CAD build for the part. Positions are in the model's coordinates, mm. A direction names the side the tool comes from. Coordinates: 2 decimals unless noted, no trailing zeros. Order: outer loops, then holes, each group sorted by start corner. A loop starts at its lowest first (then second) coordinate and runs counter-clockwise, first axis right, second up. Notation, with made-up numbers: (24.5, 81.25) - (71.5, 81.25) arc R17 ccw to (71.5, 110.25) - close; hole circle Ø10 at (80, 78.25). An arc over 180 degrees is marked (long way). Write each question's results on one line, items separated by ' | '. Start each with the question number.
Q1. Band-saw the part on B-B, the plane x = 60.5. Write the cut outline in (y, z) (3 decimals).
Q2. Pin check, flat tips, straight feed: P1, Ø1, axis at x = 22, z = 11, coming from the +Y side; P2, Ø2.5, axis at x = -77.08, y = -71.12, coming from the -Z side; P3, Ø6, axis at y = 8.5, z = 13.5, coming from the -X side. Stop position of each tip, or through.
Q3. Pull direction Y, two halves, no side cores. Call faces 5 (the flat face through (-2, 69.215, 9)), 6 (the flat face through (-2, 76.2, 4)), 7 (the flat face through (-2, -69.215, 9)), 8 (the flat face through (133.35, -1, 4)): released by +Y, released by -Y, zero draft, split by the parting line, or undercut.
Q4. Band-saw the part on A-A, the plane y = 1. Write the cut outline in (x, z) (3 decimals), then the cut area to 3 significant figures.
Q5. Wall check: probe 1 along Y at (x, z) = (-26, 6.25) (3 decimals); probe 2 along X at (y, z) = (0.5, 8.25) (3 decimals); probe 3 along Y at (x, z) = (53.5, 6.5) (3 decimals). Give the ranges that are in metal, low to high.
Q6. Which spindle directions (+Z, -Z, +X, -X, +Y, -Y) get a long thin tool onto all of the face, cutting with end or side? Do faces 1 (the flat face through (-2, 73.152, 13)), 2 (the flat face through (-2, -73.152, 13)), 3 (the flat face through (130.302, -1, 13)), 4 (the flat face through (-126.365, -1, 9)). Say none if no direction does.
```python
from build123d import *

# Parameters (mm, degrees)
F0_W      = 266.7
F0_H      = 152.4
F0_W_2    = 252.73
F0_H_2    = 138.43
F1_DEPTH  = 17.78
F2_W      = 266.7
F2_H      = 152.4
F2_W_2    = 260.604
F2_H_2    = 146.304
F3_DEPTH  = 8.89
F4_W      = 263.4996
F4_H      = 149.1996
F4_W_2    = 260.35
F4_H_2    = 146.05
F5_DEPTH  = 1.27
F6_R      = 0.762
F7_R      = 1.905
F8_R      = 1.4986
F9_DEPTH  = 8.128
F10_R     = 1.4224
F11_DEPTH = 25.4


with BuildPart() as f1:
    # F0 (on Top) → F1 (new body)
    with BuildSketch(Plane.XY):
        Rectangle(F0_W, F0_H)
        Rectangle(F0_W_2, F0_H_2, mode=Mode.SUBTRACT)
    extrude(amount=F1_DEPTH)

    # F2 (on face) → F3 (cut)
    with BuildSketch(Plane.XY.offset(17.78)):
        Rectangle(F2_W, F2_H)
        Rectangle(F2_W_2, F2_H_2, mode=Mode.SUBTRACT)
    extrude(amount=-F3_DEPTH, mode=Mode.SUBTRACT)

    # F4 (on face) → F5 (cut)
    with BuildSketch(Plane(origin=(0, 0, 0), x_dir=(1, 0, 0), z_dir=(0, 0, -1))):
        Rectangle(F4_W, F4_H)
        Rectangle(F4_W_2, F4_H_2, mode=Mode.SUBTRACT)
    extrude(amount=-F5_DEPTH, mode=Mode.SUBTRACT)

    # F6
    f6_edges = [f1.edges().sort_by_distance(p)[0] for p in [
        (-126.365, -69.215, 8.89),
        (126.365, -69.215, 8.89),
        (126.365, 69.215, 8.89),
        (-126.365, 69.215, 8.89),
    ]]
    fillet(f6_edges, radius=F6_R)

    # F7
    f7_edges = [f1.edges().sort_by_distance(p)[0] for p in [
        (130.175, 73.025, 0.635),
        (131.7498, 74.5998, 0.635),
        (-130.175, 73.025, 0.635),
        (-131.7498, 74.5998, 0.635),
        (-130.175, -73.025, 0.635),
        (-131.7498, -74.5998, 0.635),
        (130.175, -73.025, 0.635),
        (131.7498, -74.5998, 0.635),
    ]]
    fillet(f7_edges, radius=F7_R)

    # F8 (on face) → F9 (cut)
    with BuildSketch(Plane(origin=(0, 0, 0), x_dir=(1, 0, 0), z_dir=(0, 0, -1))):
        with Locations((127.949095, -71.12)):
            Circle(F8_R)
        with Locations((128.141546, -28.642724)):
            Circle(F8_R)
        with Locations((128.34959, 17.276384)):
            Circle(F8_R)
        with Locations((-127.949095, -71.12)):
            Circle(F8_R)
        with Locations((-128.34959, 17.276384)):
            Circle(F8_R)
        with Locations((-128.141546, -28.642724)):
            Circle(F8_R)
        with Locations((76.691895, -71.12)):
            Circle(F8_R)
        with Locations((25.434695, -71.12)):
            Circle(F8_R)
        with Locations((-25.822505, -71.12)):
            Circle(F8_R)
        with Locations((-77.079705, -71.12)):
            Circle(F8_R)
        with Locations((76.691895, 71.12)):
            Circle(F8_R)
        with Locations((127.949095, 71.12)):
            Circle(F8_R)
        with Locations((-127.949095, 71.12)):
            Circle(F8_R)
        with Locations((25.434695, 71.12)):
            Circle(F8_R)
        with Locations((-77.079705, 71.12)):
            Circle(F8_R)
        with Locations((-25.822505, 71.12)):
            Circle(F8_R)
    extrude(amount=-F9_DEPTH, mode=Mode.SUBTRACT)

    # F10 (on face) → F11 (cut)
    with BuildSketch(Plane(origin=(0, 73.152, 0), x_dir=(-1, 0, 0), z_dir=(0, 1, 0))):
        with Locations((-104.902, 13.335)):
            Circle(F10_R)
        with Locations((-41.402, 13.892556)):
            Circle(F10_R)
        with Locations((104.902, 13.335)):
            Circle(F10_R)
        with Locations((41.402, 13.892556)):
            Circle(F10_R)
    extrude(amount=-F11_DEPTH, mode=Mode.SUBTRACT)


solid = f1.part
```
Results below:
1) outline: (-76.2, 0) - (-74.6, 0) - (-74.6, 1.27) - (-73.025, 1.27) - (-73.025, 0) - (-69.215, 0) - (-69.215, 17.78) - (-73.152, 17.78) - (-73.152, 8.89) - (-76.2, 8.89) - close; (69.215, 0) - (73.025, 0) - (73.025, 1.27) - (74.6, 1.27) - (74.6, 0) - (76.2, 0) - (76.2, 8.89) - (73.152, 8.89) - (73.152, 17.78) - (69.215, 17.78) - close
2) P1: stops at y = 73.15 | P2: stops at z = 8.13 | P3: stops at x = -130.3
3) face 5: undercut | face 6: released by +Y | face 7: undercut | face 8: zero draft
4) outline: (-133.35, 0) - (-131.75, 0) - (-131.75, 1.27) - (-130.175, 1.27) - (-130.175, 0) - (-126.365, 0) - (-126.365, 17.78) - (-130.302, 17.78) - (-130.302, 8.89) - (-133.35, 8.89) - close; (126.365, 0) - (130.175, 0) - (130.175, 1.27) - (131.75, 1.27) - (131.75, 0) - (133.35, 0) - (133.35, 8.89) - (130.302, 8.89) - (130.302, 17.78) - (126.365, 17.78) - close | area: 190 mm²
5) probe 1: y = -76.2 to -72.608, -69.632 to -69.215, 69.215 to 69.632, 72.608 to 76.2 | probe 2: x = -133.35 to -126.365, 126.365 to 133.35 | probe 3: y = -76.2 to -69.215, 69.215 to 76.2
6) face 1: +Z, +X, -X, +Y | face 2: +Z, +X, -X, -Y | face 3: +Z, +X, +Y, -Y | face 4: +Z, -Z
